Source: CAD feature listing. Evaluate the final solid. Frame: model axes, mm. Coordinates: 2 decimals unless noted, no trailing zeros. Write each loop counter-clockwise with the first axis right and the second up, starting at its lowest first coordinate (ties: lowest second). Pieces come first, ordered by that corner, then holes. Notation, with made-up numbers: (72, -38) -> (119, -38) arc R17 cw to (119, -22) -> close; hole circle Ø6 at (10.5, -38.75). An arc over 180 degrees is marked (long way). Write item = value, one per line.
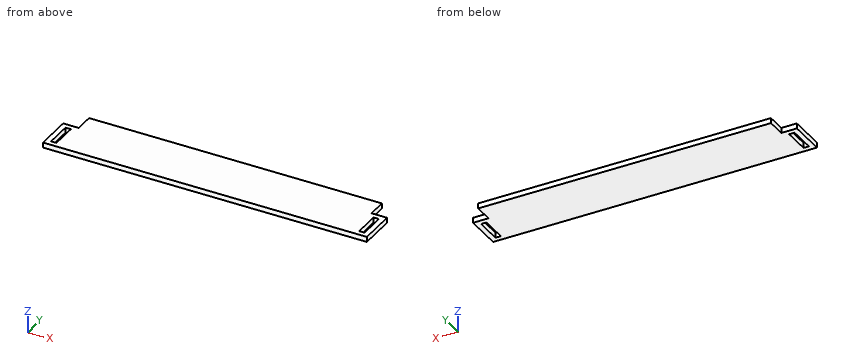
from build123d import *

# Parameters (mm, degrees)
CROQUIS1_W              = 3.123
CROQUIS1_H              = 15.13
SALIENTE_EXTRUIR1_DEPTH = 3


with BuildPart() as part:
    # Croquis1 → Saliente-Extruir1 (new body)
    with BuildSketch(Plane.XY):
        Polygon((-94, 0), (94, 0), (94, 21.123), (85, 21.123), (85, 32), (-85, 32), (-85, 21.123), (-94, 21.123), align=None)
        with Locations((-89.4385, 10.558)):
            Rectangle(CROQUIS1_W, CROQUIS1_H, mode=Mode.SUBTRACT)
        with Locations((89.4385, 10.558)):
            Rectangle(CROQUIS1_W, CROQUIS1_H, mode=Mode.SUBTRACT)
    extrude(amount=SALIENTE_EXTRUIR1_DEPTH)


solid = part.part
1) Material intervals for probe 1 along X at (y, z) = (13.5, 2.55); probe 2 along X at (y, z) = (31, 0.35), sorted ascending. Write a range as [from, to].
Answer block:
probe_1 = [-94, -91], [-87.88, 87.88], [91, 94]
probe_2 = [-85, 85]
2) Cut plane C-C, the plane y = 29.5. Output: boundary loops of the cut face in (x, z).
Answer block:
outline = (-85, 0) -> (85, 0) -> (85, 3) -> (-85, 3) -> close
3) First-contact query: pin 1 Ø1.5 at (x, z) = (-90, 1) entering from +Y; pin 2 Ø0.9 at (y, z) = (28.5, 1.5) entering from +X; pin 3 Ø0.9 at (y, z) = (29, 1) entering from -X; pin 4 Ø5 at (x, y) = (43.5, 20) entering from -Z. Flat tips, straight axial feed; report the tip coordinate or a pass-through.
Answer block:
pin_1 = 21.12
pin_2 = 85
pin_3 = -85
pin_4 = 0
4) Cut plane A-A, the plane y = 8.5. Output: boundary loops of the cut face in (x, z).
Answer block:
outline = (-94, 0) -> (-91, 0) -> (-91, 3) -> (-94, 3) -> close; (-87.88, 0) -> (87.88, 0) -> (87.88, 3) -> (-87.88, 3) -> close; (91, 0) -> (94, 0) -> (94, 3) -> (91, 3) -> close
5) Cut plane B-B, the plane z = 2.25. Output: boundary loops of the cut face in (x, y).
Answer block:
outline = (-94, 0) -> (94, 0) -> (94, 21.12) -> (85, 21.12) -> (85, 32) -> (-85, 32) -> (-85, 21.12) -> (-94, 21.12) -> close; hole (-91, 2.99) -> (-87.88, 2.99) -> (-87.88, 18.12) -> (-91, 18.12) -> close; hole (87.88, 2.99) -> (91, 2.99) -> (91, 18.12) -> (87.88, 18.12) -> close
